Check sheet for the modelled part. Datum: model origin and axes. Units: mm. A direction names the side the tool comes from. Give positions to 0.01 mm unless a question says otherwise; leave off trailing zeros. Loops run counter-clockwise (first coordinate to the right, second up) from the corner with the lowest first, then second, coordinate; pieces in that order, holes last. Notation, with made-up numbers: (48, 85.25) - (52, 85.25) arc R27 cw to (52, 107.25) - close; hole circle Ø1 at (-0.75, 14). An arc over 180 degrees is marked (long way). Answer in a Markdown table with one row per item. Add a question column.
(1) Sectioned sample at D-D on x = -3.25. Enter the section's corners in (y, z), then the cut area to 3 significant figures.
(2) Draft check along X on faces 3 (the face through (0.29, 14.23, -16.27)), 4 (the face through (-6.5, 1.7, -1)), 5 (the face through (0, 9, -18)). Enter one of: released by +X, released by -X, zero draft, split by the parting line, or undercut.
(3) Thickness scan on L1, parallel to Z at x = 0, y = 2.35; L2, parallel to Y at x = 0, z = -17.25; L3, parallel to Y at x = -4.25, z = -14.25. Record the ranges inside material, lowest first.
(4) Sectioned sample at A-A on y = 12. Enter the section's corners in (x, z).
(5) Sectioned sample at C-C on x = 0. Enter the section's corners in (y, z), then the cut area to 4 significant figures.
(6) Set-up check for faces 1 (the face through (7.5, 3, -14)), 2 (the face through (0, 9, -14.5)): record each of +Z, -Z, +X, -X, +Y, -Y from which the full face is reachable in a straight line by a thin tool's end or side.
(7) Go/stop test with flat-tipped pins: P1, Ø4, axis at x = 0, z = -5.75, coming from the -Y side; P2, Ø4, axis at x = -2.5, z = -8.5, coming from the -Y side; P3, Ø4.5, axis at x = -1, z = -7.5, coming from the +Y side. Record where each tip stops, or that it passes through.
(8) Sectioned sample at B-B on z = -5.75. Enter the section's corners in (x, y).
from build123d import *

# Parameters (mm, degrees)
SALIENTE_EXTRUIR1_DEPTH = 7.5
CROQUIS2_R              = 2.25
CORTAR_EXTRUIR1_DEPTH   = 15
CROQUIS3_R              = 2.25
CORTAR_EXTRUIR2_DEPTH   = 15
CHAFL_N1_SIZE           = 2


with BuildPart() as part:
    # Croquis1 → Saliente-Extruir1 (new body, symmetric)
    with BuildSketch(Plane(origin=(0, 0, 0), x_dir=(0, 0, -1), z_dir=(1, 0, 0))):
        Polygon((0, 0), (0, 3.5), (14.5, 3.5), (14.5, 18), (18, 18), (18, 0), align=None)
    extrude(amount=SALIENTE_EXTRUIR1_DEPTH, both=True)

    # Croquis2 → Cortar-Extruir1 (cut)
    with BuildSketch(Plane.XZ):
        with Locations((0, -5.75)):
            Circle(CROQUIS2_R)
    extrude(amount=-CORTAR_EXTRUIR1_DEPTH, mode=Mode.SUBTRACT)

    # Croquis3 → Cortar-Extruir2 (cut)
    with BuildSketch(Plane(origin=(0, 0, -18), x_dir=(-1, 0, 0), z_dir=(0, 0, -1))):
        with Locations((0, 12)):
            Circle(CROQUIS3_R)
    extrude(amount=-CORTAR_EXTRUIR2_DEPTH, mode=Mode.SUBTRACT)

    # Chaflán1
    chafl_n1_edges = [part.edges().sort_by_distance(p)[0] for p in [
        (7.5, 18, -16.25),
        (7.5, 1.75, 0),
        (-7.5, 1.75, 0),
        (-7.5, 18, -16.25),
    ]]
    chamfer(chafl_n1_edges, length=CHAFL_N1_SIZE)


solid = part.part
Reply:
| question | item | result |
|---|---|---|
| 1 | outline | (0, -18) - (18, -18) - (18, -14.5) - (3.5, -14.5) - (3.5, 0) - (0, 0) - close |
| 1 | area | 114 mm^2 |
| 2 | face 3 | undercut |
| 2 | face 4 | released by -X |
| 2 | face 5 | zero draft |
| 3 | L1 | -18 to -8, -3.5 to 0 |
| 3 | L2 | 0 to 9.75, 14.25 to 18 |
| 3 | L3 | 0 to 3.5 |
| 4 | outline | (-7.5, -18) - (-2.25, -18) - (-2.25, -14.5) - (-7.5, -14.5) - close; (2.25, -18) - (7.5, -18) - (7.5, -14.5) - (2.25, -14.5) - close |
| 5 | outline | (0, -18) - (9.75, -18) - (9.75, -14.5) - (3.5, -14.5) - (3.5, -8) - (0, -8) - close; (0, -3.5) - (3.5, -3.5) - (3.5, 0) - (0, 0) - close; (14.25, -18) - (18, -18) - (18, -14.5) - (14.25, -14.5) - close |
| 5 | area | 82.25 mm^2 |
| 6 | face 1 | +Z, -Z, +X, +Y, -Y |
| 6 | face 2 | +Z, +X, -X, +Y |
| 7 | P1 | through |
| 7 | P2 | y = 0 |
| 7 | P3 | y = 3.5 |
| 8 | outline | (-7.5, 0) - (-2.25, 0) - (-2.25, 3.5) - (-7.5, 3.5) - close; (2.25, 0) - (7.5, 0) - (7.5, 3.5) - (2.25, 3.5) - close |
